from build123d import *

# Parameters (mm, degrees)
ESBO_O2_R                = 5
CORTE_EXTRUS_O2_DEPTH    = 30
PADR_OCIRCULAR1_COUNT    = 3
ESBO_O6_R                = 6
CORTE_EXTRUS_O5_DEPTH    = 2
PADR_OCIRCULAR4_COUNT    = 3
ESBO_O9_W                = 3.998230439
ESBO_O9_H                = 6
CORTE_EXTRUS_O6_DEPTH    = 129.763348823
ESBO_O10_R               = 8.5
CORTE_EXTRUS_O7_DEPTH    = 10
PADR_OCIRCULAR5_COUNT    = 3
ESBO_O11_R               = 10
RESSALTO_EXTRUS_O1_DEPTH = 2
CORTE_EXTRUS_O9_START    = 2
ESBO_O12_R               = 8.5
CORTE_EXTRUS_O9_DEPTH    = 2
RESSALTO_EXTRUS_O2_START = 2
ESBO_O13_R               = 10
ESBO_O13_R_2             = 5
RESSALTO_EXTRUS_O2_DEPTH = 2
PADR_OCIRCULAR6_COUNT    = 3
ESBO_O14_R               = 17.5
CORTE_EXTRUS_O10_DEPTH   = 3


with BuildPart() as part:
    # Esboço1 → Revolução1 (revolve)
    with BuildSketch(Plane.XY):
        Polygon((0, 0), (48, 0), (48, 30), (40, 30), (37.866686426, 10), (32.866686426, 10), (14.223529412, 10), (9.223529412, 10), (6, 25), (0, 25), align=None)
    revolve(axis=Axis((56, 30, 0), (0, -1, 0)))

    # Esboço2 → Corte-extrusão2 (cut)
    with BuildSketch(Plane(origin=(0, 10, 0), x_dir=(1, 0, 0), z_dir=(0, 1, 0))):
        with Locations(Location((24, 0, 0), (0, 0, 180))):
            Circle(ESBO_O2_R)
    corte_extrus_o2 = extrude(amount=-CORTE_EXTRUS_O2_DEPTH, mode=Mode.SUBTRACT)

    # PadrãoCircular1: Corte-extrusão2 ×3 about axis
    padr_ocircular1_axis = Axis((56, 0, 0), (0, 1, 0))
    for i in range(1, PADR_OCIRCULAR1_COUNT):
        add(corte_extrus_o2.rotate(padr_ocircular1_axis, i * 360 / PADR_OCIRCULAR1_COUNT), mode=Mode.SUBTRACT)

    # Esboço6 → Corte-extrusão5 (cut)
    with BuildSketch(Plane.XZ):
        with Locations((24, 0)):
            Circle(ESBO_O6_R)
    corte_extrus_o5 = extrude(amount=-CORTE_EXTRUS_O5_DEPTH, mode=Mode.SUBTRACT)

    # PadrãoCircular4: Corte-extrusão5 ×3 about axis
    padr_ocircular4_axis = Axis((56, 0, 0), (0, 1, 0))
    for i in range(1, PADR_OCIRCULAR4_COUNT):
        add(corte_extrus_o5.rotate(padr_ocircular4_axis, i * 360 / PADR_OCIRCULAR4_COUNT), mode=Mode.SUBTRACT)

    # Esboço9 → Corte-extrusão6 (cut, through all)
    with BuildSketch(Plane(origin=(0, 30, 0), x_dir=(1, 0, 0), z_dir=(0, 1, 0))):
        with Locations((46.755362969, 0.391520848)):
            Rectangle(ESBO_O9_W, ESBO_O9_H)
    extrude(amount=-CORTE_EXTRUS_O6_DEPTH, mode=Mode.SUBTRACT)

    # Esboço10 → Corte-extrusão7 (cut)
    with BuildSketch(Plane(origin=(0, 10, 0), x_dir=(1, 0, 0), z_dir=(0, 1, 0))):
        with Locations(Location((40.977280539, 26.020113375, 0), (0, 0, 180))):
            Circle(ESBO_O10_R)
    corte_extrus_o7 = extrude(amount=-CORTE_EXTRUS_O7_DEPTH, mode=Mode.SUBTRACT)

    # PadrãoCircular5: Corte-extrusão7 ×3 about axis
    padr_ocircular5_axis = Axis((56, 0, 0), (0, 1, 0))
    for i in range(1, PADR_OCIRCULAR5_COUNT):
        add(corte_extrus_o7.rotate(padr_ocircular5_axis, i * 360 / PADR_OCIRCULAR5_COUNT), mode=Mode.SUBTRACT)

    # Esboço11 → Ressalto-extrusão1 (add)
    with BuildSketch(Plane(origin=(0, 10, 0), x_dir=(1, 0, 0), z_dir=(0, 1, 0))):
        with Locations(Location((40.977280539, 26.020113375, 0), (0, 0, 180))):
            Circle(ESBO_O11_R)
        with Locations(Location((86.045438923, 0, 0), (0, 0, 180))):
            Circle(ESBO_O11_R)
        with Locations(Location((40.977280539, -26.020113375, 0), (0, 0, 180))):
            Circle(ESBO_O11_R)
    extrude(amount=RESSALTO_EXTRUS_O1_DEPTH)

    # Esboço12 → Corte-extrusão9 (cut)
    with BuildSketch(Plane(origin=(0, 10, 0), x_dir=(1, 0, 0), z_dir=(0, 1, 0)).offset(CORTE_EXTRUS_O9_START)):
        with Locations(Location((40.977280539, 26.020113375, 0), (0, 0, 180))):
            Circle(ESBO_O12_R)
        with Locations(Location((40.977280539, -26.020113375, 0), (0, 0, 180))):
            Circle(ESBO_O12_R)
        with Locations(Location((86.045438923, 0, 0), (0, 0, 180))):
            Circle(ESBO_O12_R)
    extrude(amount=-CORTE_EXTRUS_O9_DEPTH, mode=Mode.SUBTRACT)

    # Esboço13 → Ressalto-extrusão2 (add)
    with BuildSketch(Plane(origin=(0, 10, 0), x_dir=(1, 0, 0), z_dir=(0, 1, 0)).offset(RESSALTO_EXTRUS_O2_START)):
        with Locations(Location((24, 0, 0), (0, 0, 180))):
            Circle(ESBO_O13_R)
        with Locations(Location((24, 0, 0), (0, 0, 180))):
            Circle(ESBO_O13_R_2, mode=Mode.SUBTRACT)
    ressalto_extrus_o2 = extrude(amount=-RESSALTO_EXTRUS_O2_DEPTH)

    # PadrãoCircular6: Corte-extrusão2, Ressalto-extrusão2 ×3 about axis
    padr_ocircular6_axis = Axis((56, 0, 0), (0, 1, 0))
    add([corte_extrus_o2.rotate(padr_ocircular6_axis, i * 360 / PADR_OCIRCULAR6_COUNT) for i in range(1, PADR_OCIRCULAR6_COUNT)], mode=Mode.SUBTRACT)
    add([ressalto_extrus_o2.rotate(padr_ocircular6_axis, i * 360 / PADR_OCIRCULAR6_COUNT) for i in range(1, PADR_OCIRCULAR6_COUNT)])

    # Esboço14 → Corte-extrusão10 (cut)
    with BuildSketch(Plane.XZ):
        with Locations((56, 0)):
            Circle(ESBO_O14_R)
    extrude(amount=-CORTE_EXTRUS_O10_DEPTH, mode=Mode.SUBTRACT)


solid = part.part
Could you check a few things on this model? Use its own coordinates, in mm. A direction names the side the tool comes from. Give positions to 0.01 mm unless a question says otherwise; leave off trailing zeros. Write each loop counter-clockwise with the first axis right and the second up, starting at its lowest first coordinate (ties: lowest second). Pieces come first, ordered by that corner, then holes. Notation, with made-up numbers: (8.5, 24.5) -> (46.5, 24.5) arc R16 cw to (46.5, 44.5) -> close; hole circle Ø10 at (45, 60). An arc over 180 degrees is marked (long way). Answer as CSV lines item,"result". Start each with the question number.
(1) If we section it at D-D, the plane y = 4.5: Write out the boundary of the cut face in (x, z).
(2) I'm going to push flat-ended pins straight in: pin 1 Ø3 at (y, z) = (17, -40) entering from -X; pin 2 Ø9.5 at (x, z) = (72, -27.71) entering from +Y; pin 3 Ø1 at (x, y) = (29.5, 5.5) entering from -Z; pin 4 Ø10 at (x, z) = (42, 22.5) entering from +Y. Where does each tip first touch, or does it pass through?
(3) If we section it at B-B, the plane x = 56: Write out the boundary of the cut face in (y, z).
(4) If we mould it in two halves opening along X, with no side actions, what happens to faces 4 (the face through (2.586, 12.325, -16.821)), 5 (the face through (76.81, 10.99, -3.83)), 6 (the face through (69, 12, -32)), 7 (the face through (35, 25, -46))? For each: +X half, -X half, draft (parallel to the pull), parting line (faces both ways), or undercut.
(5) Please list where these lines run through material, in increasing order: line 1 (Z direction, x = 28, y = 10.25); line 2 (X direction, y = 15.5, z = 0); line 3 (Y direction, x = 61.5, z = -45).
(6) If we section it at A-A, the plane y = 17.25: Write out the boundary of the cut face in (x, z).
(7) Which directions (+Z, -Z, +X, -X, +Y, -Y) give clear straight access to the entire face, cutting with the end or side of a thin tool? Please do faces 1 (the face through (74.17, 11.01, 17.95)), 2 (the face through (20, 2, 4)), 3 (the face through (44.756, 17, 0)).
(8) If we section it at C-C, the plane z = 0: Give the number of separate pieces and of enclosed holes in the cut face, and give its area (3 significant figures).
Answer list:
1,outline,"circle Ø112 at (56, 0); hole circle Ø10 at (24, 0); hole circle Ø17 at (40.98, -26.02); hole circle Ø17 at (40.98, 26.02); hole (44.76, -3.39) -> (48.75, -3.39) arc R8 ccw (long way) to (48.44, 2.61) -> (44.76, 2.61) -> close; hole circle Ø10 at (72, -27.71); hole circle Ø10 at (72, 27.71); hole circle Ø17 at (86.05, 0)"
2,pin 1,"x = 15.33"
2,pin 2,"through"
2,pin 3,"z = -49.6"
2,pin 4,"y = 12"
3,outline,"(0, -56) -> (25, -56) -> (25, -50) -> (10, -46.78) -> (10, -18.13) -> (30, -16) -> (30, -8) -> (3, -8) -> (3, -17.5) -> (0, -17.5) -> close; (0, 17.5) -> (3, 17.5) -> (3, 8) -> (30, 8) -> (30, 16) -> (10, 18.13) -> (10, 46.78) -> (25, 50) -> (25, 56) -> (0, 56) -> close"
4,face 4,"parting line"
4,face 5,"undercut"
4,face 6,"undercut"
4,face 7,"draft"
5,line 1,"-48.5 to -37.54, -9.17 to -3, 3 to 9.17, 37.54 to 48.5"
5,line 2,"0 to 8.04, 38.45 to 44.76, 64 to 73.55, 103.96 to 112"
5,line 3,"0 to 10"
6,outline,"circle Ø112 at (56, 0); circle Ø34.72 at (56, 0); hole circle Ø96.67 at (56, 0); hole (44.76, -3.39) -> (48.75, -3.39) arc R8 ccw (long way) to (48.44, 2.61) -> (44.76, 2.61) -> close"
7,face 1,"+Y"
7,face 2,"-Y"
7,face 3,"+Y, -Y"
8,separate pieces,"4"
8,enclosed holes,"0"
8,area,"1,160 mm^2"
